Could you check a few things on this model? Use its own coordinates, in mm. A direction names the side the tool comes from. Coordinates: 2 decimals unless noted, no trailing zeros. Order: outer loops, then holes, each group sorted by start corner. A loop starts at its lowest first (then second) coordinate and runs counter-clockwise, first axis right, second up. Notation, with made-up numbers: (4, 13.5) -> (53, 13.5) arc R27 cw to (53, 46.5) -> close; hole circle Ø10 at (-5.75, -33.75). An arc over 180 degrees is marked (long way). Use a Markdown table: item, result. Add a question column.
1) Thinking about a two-plate mould opening in Z: for faces 1 (the cylindrical face through (3.99, -1.07, -26.9)), 2 (the flat face through (-4, -6, 28.5)), 3 (the cylindrical face through (4.01, -0.36, -27.6)), which applies, +Z half, -Z half, draft (parallel to the pull), parting line (faces both ways), or undercut?
2) Will these pins go through, and if not, where does the flat tip stop? pin 1 Ø10 at (x, z) = (6, 21) entering from -Y; pin 2 Ø0.6 at (x, z) = (4, 24) entering from +Y; pin 3 Ø1 at (x, y) = (-6, -6) entering from +Z; pin 4 Ø1.5 at (y, z) = (-5, 26.5) entering from -X.
3) Which directions (+Z, -Z, +X, -X, +Y, -Y) give clear straight access to the entire face, cutting with the end or side of a thin tool? Please do faces 4 (the flat face through (-4, 0.5, -25)), 5 (the flat face through (-3, -3, 28)), 6 (the flat face through (4, -0.5, 25)), 7 (the flat face through (-5, -3, -28)).
4) If we section it at B-B (y = -3.5): Write out the boundary of the cut face in (x, z).
5) If we section it at A-A (x = 3.75): Write out the boundary of the cut face in (y, z).
6) If we section it at C-C (z = 13): Write out the boundary of the cut face in (x, y), plus the area to 3 significant figures.
7) If we section it at D-D (y = 2.75): Write out the boundary of the cut face in (x, z).
8) If I drill on L1, parallel to Z at x = 3.25, y = -6.5; L2, parallel to Z at x = 2.5, y = -3.5; L3, parallel to Z at x = 9, y = -4.75, over which ranges is the centre line in solid material (lowest first)? Write a range as [from, to].
```python
from build123d import *

# Parameters (mm, degrees)
EXTRUDE1_DEPTH          = 23
EXTRUDE2_DEPTH          = 23.5
SKETCH6_W               = 2
SKETCH6_H               = 1
MIRROR2_COPY_1_SKETCH_W = 2
MIRROR2_COPY_1_SKETCH_H = 1


with BuildPart() as part:
    # Sketch1 → Extrude1 (new, symmetric)
    with BuildSketch(Plane.XY):
        with BuildLine():
            Line((-4.5, 8), (4.5, 8))
            ThreePointArc((4.5, 8), (12.5, 0), (4.5, -8))
            Line((4.5, -8), (-4.5, -8))
            ThreePointArc((-4.5, -8), (-12.5, 0), (-4.5, 8))
        make_face()
    extrude(amount=EXTRUDE1_DEPTH, both=True)

    # Sketch2 → Extrude2 (add, symmetric)
    with BuildSketch(Plane.XY):
        with BuildLine():
            Line((-4.5, -5), (4.5, -5))
            ThreePointArc((4.5, -5), (9.5, 0), (4.5, 5))
            Line((4.5, 5), (-4.5, 5))
            ThreePointArc((-4.5, 5), (-9.5, 0), (-4.5, -5))
        make_face()
    extrude(amount=EXTRUDE2_DEPTH, both=True)

    # Sweep1: sweep along a path in Sketch3
    with BuildLine(Plane(origin=(-4, 0, 0), x_dir=(0, 0, -1), z_dir=(1, 0, 0))) as sweep1_path:
        Line((0, 0), (-25.5, 0))
        ThreePointArc((-25.5, 0), (-27.267766953, -0.732233047), (-28, -2.5))
        Line((-28, -2.5), (-28, -10))
    # Sketch6 → Sweep1 (sweep)
    with BuildSketch(Plane.XY):
        with Locations((-4, 0)):
            Rectangle(SKETCH6_W, SKETCH6_H)
    sweep1 = sweep(path=sweep1_path.line)

    # Mirror1: Sweep1 across plane
    add(sweep1.mirror(Plane(origin=(0, 0, 0), x_dir=(0, 0, 1), z_dir=(1, 0, 0))))

    # Mirror2: Sweep1 across plane
    add(sweep1.mirror(Plane.XY))

    # Mirror2 copy 1: sweep along a path in Mirror2 copy 1 path
    with BuildLine(Plane.ZY.offset(-4)) as mirror2_copy_1_path:
        Line((0, 0), (-25.5, 0))
        ThreePointArc((-25.5, 0), (-27.267766953, -0.732233047), (-28, -2.5))
        Line((-28, -2.5), (-28, -10))
    # Mirror2 copy 1 sketch → Mirror2 copy 1 (sweep)
    with BuildSketch(Plane(origin=(0, 0, 0), x_dir=(-1, 0, 0), z_dir=(0, 0, -1))):
        with Locations((-4, 0)):
            Rectangle(MIRROR2_COPY_1_SKETCH_W, MIRROR2_COPY_1_SKETCH_H)
    sweep(path=mirror2_copy_1_path.line)


solid = part.part
```
Answer sheet:
| question | item | result |
|---|---|---|
| 1 | face 1 | undercut |
| 1 | face 2 | +Z half |
| 1 | face 3 | -Z half |
| 2 | pin 1 | y = -8 |
| 2 | pin 2 | y = 0.5 |
| 2 | pin 3 | z = 23 |
| 2 | pin 4 | through |
| 3 | face 4 | -Z, +X, -X, +Y |
| 3 | face 5 | +Z, +Y, -Y |
| 3 | face 6 | +X, -X, -Y |
| 3 | face 7 | -Z, -X, +Y, -Y |
| 4 | outline | (-11.69, -23) -> (-8.07, -23) -> (-8.07, -23.5) -> (8.07, -23.5) -> (8.07, -23) -> (11.69, -23) -> (11.69, 23) -> (8.07, 23) -> (8.07, 23.5) -> (-8.07, 23.5) -> (-8.07, 23) -> (-11.69, 23) -> close; (-5, -28.5) -> (-3, -28.5) -> (-3, -27.5) -> (-5, -27.5) -> close; (-5, 27.5) -> (-3, 27.5) -> (-3, 28.5) -> (-5, 28.5) -> close; (3, -28.5) -> (5, -28.5) -> (5, -27.5) -> (3, -27.5) -> close; (3, 27.5) -> (5, 27.5) -> (5, 28.5) -> (3, 28.5) -> close |
| 5 | outline | (-10, -28.5) -> (-2.5, -28.5) arc R3 ccw to (0.5, -25.5) -> (0.5, -23.5) -> (5, -23.5) -> (5, -23) -> (8, -23) -> (8, 23) -> (5, 23) -> (5, 23.5) -> (0.5, 23.5) -> (0.5, 25.5) arc R3 ccw to (-2.5, 28.5) -> (-10, 28.5) -> (-10, 27.5) -> (-2.5, 27.5) arc R2 cw to (-0.5, 25.5) -> (-0.5, 23.5) -> (-5, 23.5) -> (-5, 23) -> (-8, 23) -> (-8, -23) -> (-5, -23) -> (-5, -23.5) -> (-0.5, -23.5) -> (-0.5, -25.5) arc R2 cw to (-2.5, -27.5) -> (-10, -27.5) -> close |
| 6 | outline | (-4.5, -8) -> (4.5, -8) arc R8 ccw to (4.5, 8) -> (-4.5, 8) arc R8 ccw to start |
| 6 | area | 345 mm2 |
| 7 | outline | (-12.01, -23) -> (-8.68, -23) -> (-8.68, -23.5) -> (8.68, -23.5) -> (8.68, -23) -> (12.01, -23) -> (12.01, 23) -> (8.68, 23) -> (8.68, 23.5) -> (-8.68, 23.5) -> (-8.68, 23) -> (-12.01, 23) -> close |
| 8 | L1 | [-28.5, -27.5], [-23, 23], [27.5, 28.5] |
| 8 | L2 | [-23.5, 23.5] |
| 8 | L3 | [-23, 23] |
